from build123d import *

# Parameters (mm, degrees)
SKETCH_1_W          = 32
SKETCH_1_H          = 34
EXTRUDE_1_DEPTH     = 3.5
EXTRUDE_START       = -2.5
SKETCH_1_30_W       = 32
SKETCH_1_30_H       = 34
EXTRUDE_2_DEPTH     = 2.5
EXTRUDE_START_2     = -4.5
SKETCH_1_31_W       = 32
SKETCH_1_31_H       = 34
SKETCH_1_31_R       = 5
EXTRUDE_3_DEPTH     = 2
SKETCH_1_32_W       = 32
SKETCH_1_32_H       = 34
SKETCH_1_32_R       = 3.1
EXTRUDE_4_DEPTH     = 2.7
SKETCH_2_R          = 1.5
CUT_EXTRUDE_1_DEPTH = 32.693690224
SKETCH_2_3_R        = 2.25
CUT_EXTRUDE_2_DEPTH = 8.7
SKETCH_1_33_R       = 1.15
CUT_EXTRUDE_3_DEPTH = 4
SKETCH_3_W          = 5.5
SKETCH_3_H          = 13
SKETCH_3_R          = 1.5
SKETCH_3_W_2        = 8
SKETCH_3_W_3        = 5
SKETCH_3_H_2        = 3
EXTRUDE_5_DEPTH     = 2
SKETCH_1_34_R       = 1.15
CUT_EXTRUDE_4_DEPTH = 5.2
CUT_EXTRUDE_START   = 3.5
SKETCH_1_37_R       = 1.15
CUT_EXTRUDE_6_DEPTH = 2


with BuildPart() as part:
    # 草图1 → 凸台-拉伸1 (new body)
    with BuildSketch(Plane(origin=(0, 0, 0), x_dir=(1, 0, 0), z_dir=(0, 1, 0))):
        with Locations((3, 6)):
            Rectangle(SKETCH_1_W, SKETCH_1_H)
        with BuildLine():
            ThreePointArc((13.731280316, -4.4612147), (-3.554893366, -4.816108921), (4.687954327, 10.382351934))
            ThreePointArc((4.687954327, 10.382351934), (8.931780662, 14.858222386), (10.315634647, 8.847529713))
            ThreePointArc((10.315634647, 8.847529713), (12.64747139, 6.812247403), (14.245257691, 4.161414399))
            ThreePointArc((14.245257691, 4.161414399), (16.464642722, -0.297511749), (13.731280316, -4.4612147))
        make_face(mode=Mode.SUBTRACT)
    extrude(amount=EXTRUDE_1_DEPTH)

    # 草图1<30> → 凸台-拉伸2 (add)
    with BuildSketch(Plane(origin=(0, 0, 0), x_dir=(1, 0, 0), z_dir=(0, 1, 0)).offset(EXTRUDE_START)):
        with Locations((3, 6)):
            Rectangle(SKETCH_1_30_W, SKETCH_1_30_H)
        with BuildLine():
            ThreePointArc((7.408784414, 2.911712865), (16.464642722, -0.297511749), (7.091673359, -2.408231444))
            ThreePointArc((7.091673359, -2.408231444), (1.49122024, 0.595023498), (7.408784414, 2.911712865))
        make_face(mode=Mode.SUBTRACT)
    extrude(amount=EXTRUDE_2_DEPTH)

    # 草图1<31> → 凸台-拉伸3 (add)
    with BuildSketch(Plane(origin=(0, 0, 0), x_dir=(1, 0, 0), z_dir=(0, 1, 0)).offset(EXTRUDE_START_2)):
        with Locations((3, 6)):
            Rectangle(SKETCH_1_31_W, SKETCH_1_31_H)
        with Locations(Location((11.473501894, 0, 0), (0, 0, 56.333964125))):
            Circle(SKETCH_1_31_R, mode=Mode.SUBTRACT)
    extrude(amount=EXTRUDE_3_DEPTH)

    # 草图1<32> → 凸台-拉伸4 (add)
    with BuildSketch(Plane(origin=(0, 0, 0), x_dir=(1, 0, 0), z_dir=(0, 1, 0)).offset(EXTRUDE_START_2)):
        with Locations((3, 6)):
            Rectangle(SKETCH_1_32_W, SKETCH_1_32_H)
        with Locations(Location((11.473501894, 0, 0), (0, 0, 270))):
            Circle(SKETCH_1_32_R, mode=Mode.SUBTRACT)
    extrude(amount=-EXTRUDE_4_DEPTH)

    # 草图2 → 切除-拉伸1 (cut, through all)
    with BuildSketch(Plane.XZ.offset(7.2)):
        with Locations(Location((-8, -18, 0), (0, 0, 270))):
            Circle(SKETCH_2_R)
        with Locations(Location((-7, -6, 0), (0, 0, 270))):
            Circle(SKETCH_2_R)
    extrude(amount=-CUT_EXTRUDE_1_DEPTH, mode=Mode.SUBTRACT)

    # 草图2<3> → 切除-拉伸2 (cut)
    with BuildSketch(Plane.XZ.offset(7.2)):
        with Locations(Location((-8, -18, 0), (0, 0, 270))):
            Circle(SKETCH_2_3_R)
        with Locations(Location((-7, -6, 0), (0, 0, 270))):
            Circle(SKETCH_2_3_R)
    extrude(amount=-CUT_EXTRUDE_2_DEPTH, mode=Mode.SUBTRACT)

    # 草图1<33> → 切除-拉伸3 (cut)
    with BuildSketch(Plane(origin=(0, 0, 0), x_dir=(1, 0, 0), z_dir=(0, 1, 0))):
        with Locations(Location((-3.489130435, 11.48154906, 0), (0, 0, 270))):
            Circle(SKETCH_1_33_R)
        with Locations(Location((8.010869565, 11.48154906, 0), (0, 0, 270))):
            Circle(SKETCH_1_33_R)
    extrude(amount=-CUT_EXTRUDE_3_DEPTH, mode=Mode.SUBTRACT)

    # 草图3 → 凸台-拉伸5 (add)
    # profile 1 of 4: a face of its own
    with BuildSketch(Plane.XZ.offset(7.2)):
        with Locations((-10.25, 17.5)):
            Rectangle(SKETCH_3_W, SKETCH_3_H)
        with Locations(Location((-10.12152848, 20.714718626, 0), (0, 0, 270))):
            Circle(SKETCH_3_R, mode=Mode.SUBTRACT)
    # profile 2 of 4: a face of its own
    with BuildSketch(Plane.XZ.offset(7.2)):
        with Locations((15, 17.5)):
            Rectangle(SKETCH_3_W_2, SKETCH_3_H)
        with Locations(Location((15.05833067, 20.714718626, 0), (0, 0, 270))):
            Circle(SKETCH_3_R, mode=Mode.SUBTRACT)
    # profile 3 of 4: a face of its own
    with BuildSketch(Plane.XZ.offset(7.2)):
        Polygon((19, -23), (18, -23), (18, -36), (24, -36), (24, -23), align=None)
        with Locations(Location((21.021229109, -33.234018716, 0), (0, 0, 270))):
            Circle(SKETCH_3_R, mode=Mode.SUBTRACT)
    # profile 4 of 4: a face of its own
    with BuildSketch(Plane.XZ.offset(7.2)):
        with Locations((21.5, -21.5)):
            Rectangle(SKETCH_3_W_3, SKETCH_3_H_2)
    extrude(amount=-EXTRUDE_5_DEPTH)

    # 草图1<34> → 切除-拉伸4 (cut)
    with BuildSketch(Plane(origin=(0, 0, 0), x_dir=(1, 0, 0), z_dir=(0, 1, 0))):
        with Locations(Location((4.985018819, 0.386765274, 0), (0, 0, 90))):
            Circle(SKETCH_1_34_R)
    extrude(amount=-CUT_EXTRUDE_4_DEPTH, mode=Mode.SUBTRACT)

    # 草图1<37> → 切除-拉伸6 (cut)
    with BuildSketch(Plane(origin=(0, 0, 0), x_dir=(1, 0, 0), z_dir=(0, 1, 0)).offset(CUT_EXTRUDE_START)):
        with Locations(Location((-3.489130435, 11.48154906, 0), (0, 0, 90))):
            Circle(SKETCH_1_37_R)
    extrude(amount=-CUT_EXTRUDE_6_DEPTH, mode=Mode.SUBTRACT)


solid = part.part
Model file for the job. Use its own axes, mm. A direction names the side the tool comes from. Round coordinates to 2 decimals unless told otherwise and drop trailing zeros. Loops run counter-clockwise (first coordinate to the right, second up) from the corner with the lowest first, then second, coordinate; pieces in that order, holes last.
1. Band-saw the part on B-B, the plane y = -1. List the corners of the cut face in (x, z), and give its area (3 significant figures).
Check values:
outline: (-13, -23) - (19, -23) - (19, 11) - (-13, 11) - close; hole circle Ø4.5 at (-8, -18); hole circle Ø4.5 at (-7, -6); hole circle Ø2.3 at (-3.49, -11.48); hole circle Ø2.3 at (8.01, -11.48); hole (7.09, 2.41) arc R3.5 ccw (long way) to (7.41, -2.91) arc R5 ccw (long way) to start
area: 938 mm2
2. Wall check: probe 1 along Z at (x, y) = (-7.5, 3.25); probe 2 along Y at (x, z) = (-1.5, -3.5); probe 3 along Z at (x, y) = (12, -0.25). Give the ranges that are in metal, low to high.
Check values:
probe 1: z = -23 to -19.41, -16.59 to -7.41, -4.59 to 11
probe 2: y = -7.2 to 0
probe 3: z = -23 to -4.97, 4.97 to 11
3. Mould opens along Y. For faces 1 (the cylindrical face through (-7.93, 2.49, -16.5)), 2 (the flat face through (-3, -4, -11)), 3 (the flat face through (-10, -5.2, 18)) say: +Y half, -Y half, draft (parallel to the pull), parting line (faces both ways), or undercut.
Check values:
face 1: draft
face 2: undercut
face 3: +Y half
4. Band-saw the part on D-D, the plane z = -18. List the corners of the cut face in (x, y), and give its area (3 significant figures).
Check values:
outline: (-13, -7.2) - (-10.25, -7.2) - (-10.25, 1.5) - (-9.5, 1.5) - (-9.5, 3.5) - (-13, 3.5) - close; (-6.5, 1.5) - (-5.75, 1.5) - (-5.75, -7.2) - (19, -7.2) - (19, 3.5) - (-6.5, 3.5) - close
area: 297 mm2
5. Band-saw the part on C-C, the plane z = -11.5. List the corners of the cut face in (x, y), and give its area (3 significant figures).
Check values:
outline: (-13, -7.2) - (19, -7.2) - (19, 3.5) - (11.51, 3.5) - (11.51, 0) - (9.16, 0) - (9.16, -4) - (6.86, -4) - (6.86, 0) - (4.51, 0) - (4.51, 3.5) - (-2.34, 3.5) - (-2.34, 1.5) - (-4.64, 1.5) - (-4.64, 3.5) - (-13, 3.5) - close; hole (-4.64, -4) - (-2.34, -4) - (-2.34, 0) - (-4.64, 0) - close
area: 295 mm2
6. Drop flat-ended pins along their axis: P1, Ø0.6, axis at x = 21.5, y = -6.5, coming from the +Z side; P2, Ø3, axis at x = -10.5, z = 16.5, coming from the +Y side; P3, Ø2.5, axis at x = -7, z = -6, coming from the -Y side; P4, Ø3.5, axis at x = -7, z = -6, coming from the -Y side. Give the stop position or say it passes through.
Check values:
P1: stops at z = -20
P2: stops at y = -5.2
P3: passes through
P4: stops at y = 1.5
7. Band-saw the part on A-A, the plane z = 14.5. List the corners of the cut face in (x, y), and give its area (3 significant figures).
Check values:
outline: (-13, -7.2) - (-7.5, -7.2) - (-7.5, -5.2) - (-13, -5.2) - close; (11, -7.2) - (19, -7.2) - (19, -5.2) - (11, -5.2) - close
area: 27.0 mm2
8. Tool access for faces 4 (the flat face through (15, -5.2, 18)), 5 (the flat face through (3.7, -2.5, -1.2)), 6 (the flat face through (21, -6, -20)), 7 (the flat face through (-8, 1.5, -16)): list every direction of +Z, -Z, +X, -X, +Y, -Y with a clear straight run to the whole face (end or side of a thin tool).
Check values:
face 4: +Z, +X, -X, +Y
face 5: +Y
face 6: +Z, +X, +Y, -Y
face 7: -Y
